Source: CAD feature listing. Evaluate the final solid. Frame: model axes, mm. A direction names the side the tool comes from. Give positions to 0.01 mm unless a question says otherwise; leave off trailing zeros. Loops run counter-clockwise (first coordinate to the right, second up) from the corner with the lowest first, then second, coordinate; pieces in that order, holes last. Notation, with made-up numbers: M 8.25,-19 L 36.25,-19 A33 cw 36.25,16 Z; hole C -37.75,79.5 d3. An arc over 180 degrees is marked long. Answer in a Markdown table with one row per item.
```python
from build123d import *

# Parameters (mm, degrees)
F0_W          = 101.6
F0_H          = 95.25
F1_DEPTH      = 38.1
F1_DEPTH_BACK = 38.1
F2_R          = 19.05
F3_DEPTH      = 25.4
F4_W          = 95.25
F4_H          = 76.2
F5_DEPTH      = 12.7


with BuildPart() as f1:
    # F0 (on Top) → F1 (new body, two sides)
    with BuildSketch(Plane.XY) as f1_sk:
        with Locations((50.8, 47.625)):
            Rectangle(F0_W, F0_H)
    extrude(amount=F1_DEPTH)
    extrude(f1_sk.sketch, amount=-F1_DEPTH_BACK)

    # F2 (on face) → F3 (join)
    with BuildSketch(Plane.XY.offset(38.1)):
        with Locations((44.45, 53.34)):
            Circle(F2_R)
    extrude(amount=F3_DEPTH)

    # F4 (on face) → F5 (join)
    with BuildSketch(Plane.YZ.offset(101.6)):
        with Locations((47.625, 0)):
            Rectangle(F4_W, F4_H)
        with BuildLine():
            ThreePointArc((46.342392, 22.897961), (50.403336, 31.381813), (58.886788, 27.320033))
            Line((58.886788, 27.320033), (77.276431, -24.863524))
            ThreePointArc((77.276431, -24.863524), (77.291216, -24.905044), (77.305728, -24.94666))
            ThreePointArc((77.305728, -24.94666), (73.828073, -33.213667), (65.22953, -30.663658))
            ThreePointArc((65.22953, -30.663658), (64.613677, -29.374051), (64.284402, -27.983389))
            Line((64.284402, -27.983389), (46.342392, 22.897961))
        make_face(mode=Mode.SUBTRACT)
    extrude(amount=F5_DEPTH)


solid = f1.part
```
1) Section D-D, the plane x = 71. Return loops of the section in (y, z).
Reply:
| item | result |
|---|---|
| outline | M 0,-38.1 L 95.25,-38.1 L 95.25,38.1 L 0,38.1 Z |
2) Pull-direction query (Y, two-part tool) for faces 1 (the cylindrical face through (107.861, 50.266, 31.332)), 2 (the flat face through (101.6, 62, -1)), 3 (the flat face through (56, 0, -1)), 4 (the flat face through (56, 95.25, -1)); classes: released by +Y, released by -Y, zero draft, split by the parting line, or undercut.
Reply:
| item | result |
|---|---|
| face 1 | undercut |
| face 2 | undercut |
| face 3 | released by -Y |
| face 4 | released by +Y |
3) Section A-A, the plane x = 44.45. Return loops of the section in (y, z).
Reply:
| item | result |
|---|---|
| outline | M 0,-38.1 L 95.25,-38.1 L 95.25,38.1 L 72.39,38.1 L 72.39,63.5 L 34.29,63.5 L 34.29,38.1 L 0,38.1 Z |
4) Material intervals for L1, parallel to Z at x = 96.5, y = 59; L2, parallel to X at y = 43.5, z = 59.5; L3, parallel to Y at x = 51, z = 57.5, sorted ascending.
Reply:
| item | result |
|---|---|
| L1 | z = -38.1 to 38.1 |
| L2 | x = 28.14 to 60.76 |
| L3 | y = 35.45 to 71.23 |
5) Section C-C, the plane y = 61. Return loops of the section in (x, z), then the cut area to 3 significant figures.
Reply:
| item | result |
|---|---|
| outline | M 0,-38.1 L 114.3,-38.1 L 114.3,-18.67 L 101.6,-18.67 L 101.6,21.32 L 114.3,21.32 L 114.3,38.1 L 61.89,38.1 L 61.89,63.5 L 27.01,63.5 L 27.01,38.1 L 0,38.1 Z |
| area | 9,090 mm² |
6) Pin query (flat end, axial travel): pin 1 Ø6 at (x, y) = (25.5, 15.5) entering from +Z. Return the tip coordinate at first contact, or that it passes through.
Reply:
| item | result |
|---|---|
| pin 1 | stops at z = 38.1 |
7) Section B-B, the plane z = -21.5. Return loops of the section in (x, y), then the cut area to 3 significant figures.
Reply:
| item | result |
|---|---|
| outline | M 0,0 L 114.3,0 L 114.3,62 L 101.6,62 L 101.6,76.09 L 114.3,76.09 L 114.3,95.25 L 0,95.25 Z |
| area | 10,700 mm² |
8) Set-up query: faces 5 (the cylindrical face through (40.32, 34.743, 50.622)), 6 (the flat face through (56, 47, -38.1)), 7 (the flat face through (107.86, 55.44, -2.9)). Return all of +Z, -Z, +X, -X, +Y, -Y with unobstructed straight access to the full face (end or side cutting, diameter ignored); none if empty.
Reply:
| item | result |
|---|---|
| face 5 | +Z |
| face 6 | -Z, +X, -X, +Y, -Y |
| face 7 | +X |
